Can you work these out from the model? Positions are in its coordinate system, mm. A direction names the side the tool comes from. Give positions to 0.01 mm unless a question says otherwise; leave off trailing zeros. Loops run counter-clockwise (first coordinate to the right, second up) from the corner with the lowest first, then second, coordinate; pieces in that order, holes last. Notation, with made-up numbers: (28, 26) -> (74, 26) arc R21 cw to (74, 48) -> close; hole circle Ø8 at (79, 48.5). An arc over 180 degrees is marked (long way). Use CSV: the item, a comma, the result in double quotes.
Autodesk Inventor part; units mm, degrees
ref_plane "YZ Plane" through (0, 0, 0) normal (1, 0, 0) x (0, 1, 0)
ref_plane "XZ Plane" through (0, 0, 0) normal (0, 1, 0) x (-1, 0, 0)
ref_plane "XY Plane" through (0, 0, 0) normal (0, 0, 1) x (1, 0, 0)
sketch "Sketch1" plane through (0, 0, 0) normal (0, 1, 0) x (-1, 0, 0)
  line L0 (0, 0) -> (177.8, 0)
  line L1 (177.8, 0) -> (177.8, -508)
  line L2 (177.8, -508) -> (0, -508)
  line L3 (0, -508) -> (0, 0)
  line L4 (11.987, 4.1955) -> (189.787, -503.8045)
  line L5 (-11.987, -4.1955) -> (165.813, -512.1955)
  line L6 (0, -38.444) -> (164.3446, -508)
  line L7 (177.8, -469.556) -> (13.4554, 0)
  line L8 (-11.987, -4.1955) -> (11.987, 4.1955)
  line L9 (189.787, -503.8045) -> (165.813, -512.1955)
  line L10 (0, 0) -> (2.0977, -5.9935)
  circle A0 centre (2.0977, -5.9935) radius 2.032
  line L11 (2.0977, -5.9935) -> (10.4886, -29.9675)
  circle A1 centre (10.4886, -29.9675) radius 2.032
  line L12 (10.4886, -29.9675) -> (18.8795, -53.9415)
  circle A2 centre (18.8795, -53.9415) radius 2.032
  line L13 (18.8795, -53.9415) -> (27.2704, -77.9155)
  circle A3 centre (27.2704, -77.9155) radius 2.032
  line L14 (27.2704, -77.9155) -> (35.6613, -101.8895)
  circle A4 centre (35.6613, -101.8895) radius 2.032
  line L15 (35.6613, -101.8895) -> (177.8, -508)
  line L16 (27.2704, -77.9155) -> (35.6613, -101.8895)
  circle A5 centre (35.6613, -101.8895) radius 2.032
  line L17 (35.6613, -101.8895) -> (44.0522, -125.8635)
  circle A6 centre (44.0522, -125.8635) radius 2.032
  line L18 (35.6613, -101.8895) -> (44.0522, -125.8635)
  circle A7 centre (44.0522, -125.8635) radius 2.032
  line L19 (44.0522, -125.8635) -> (52.4431, -149.8375)
  circle A8 centre (52.4431, -149.8375) radius 2.032
  line L20 (44.0522, -125.8635) -> (52.4431, -149.8375)
  circle A9 centre (52.4431, -149.8375) radius 2.032
  line L21 (52.4431, -149.8375) -> (60.834, -173.8115)
  circle A10 centre (60.834, -173.8115) radius 2.032
  line L22 (52.4431, -149.8375) -> (60.834, -173.8115)
  circle A11 centre (60.834, -173.8115) radius 2.032
  line L23 (60.834, -173.8115) -> (69.2249, -197.7855)
  circle A12 centre (69.2249, -197.7855) radius 2.032
  line L24 (60.834, -173.8115) -> (69.2249, -197.7855)
  circle A13 centre (69.2249, -197.7855) radius 2.032
  line L25 (69.2249, -197.7855) -> (77.6158, -221.7595)
  circle A14 centre (77.6158, -221.7595) radius 2.032
  line L26 (69.2249, -197.7855) -> (77.6158, -221.7595)
  circle A15 centre (77.6158, -221.7595) radius 2.032
  line L27 (77.6158, -221.7595) -> (86.0067, -245.7335)
  circle A16 centre (86.0067, -245.7335) radius 2.032
  line L28 (77.6158, -221.7595) -> (86.0067, -245.7335)
  circle A17 centre (86.0067, -245.7335) radius 2.032
  line L29 (86.0067, -245.7335) -> (94.3976, -269.7075)
  circle A18 centre (94.3976, -269.7075) radius 2.032
  line L30 (86.0067, -245.7335) -> (94.3976, -269.7075)
  circle A19 centre (94.3976, -269.7075) radius 2.032
  line L31 (94.3976, -269.7075) -> (102.7885, -293.6815)
  circle A20 centre (102.7885, -293.6815) radius 2.032
  line L32 (94.3976, -269.7075) -> (102.7885, -293.6815)
  circle A21 centre (102.7885, -293.6815) radius 2.032
  line L33 (102.7885, -293.6815) -> (111.1794, -317.6555)
  circle A22 centre (111.1794, -317.6555) radius 2.032
  line L34 (102.7885, -293.6815) -> (111.1794, -317.6555)
  circle A23 centre (111.1794, -317.6555) radius 2.032
  line L35 (111.1794, -317.6555) -> (119.5703, -341.6295)
  circle A24 centre (119.5703, -341.6295) radius 2.032
  line L36 (111.1794, -317.6555) -> (119.5703, -341.6295)
  circle A25 centre (119.5703, -341.6295) radius 2.032
  line L37 (119.5703, -341.6295) -> (127.9612, -365.6035)
  circle A26 centre (127.9612, -365.6035) radius 2.032
  line L38 (119.5703, -341.6295) -> (127.9612, -365.6035)
  circle A27 centre (127.9612, -365.6035) radius 2.032
  line L39 (127.9612, -365.6035) -> (136.3521, -389.5775)
  circle A28 centre (136.3521, -389.5775) radius 2.032
  line L40 (127.9612, -365.6035) -> (136.3521, -389.5775)
  circle A29 centre (136.3521, -389.5775) radius 2.032
  line L41 (136.3521, -389.5775) -> (144.743, -413.5515)
  circle A30 centre (144.743, -413.5515) radius 2.032
  line L42 (136.3521, -389.5775) -> (144.743, -413.5515)
  circle A31 centre (144.743, -413.5515) radius 2.032
  line L43 (144.743, -413.5515) -> (153.1339, -437.5255)
  circle A32 centre (153.1339, -437.5255) radius 2.032
  line L44 (144.743, -413.5515) -> (153.1339, -437.5255)
  circle A33 centre (153.1339, -437.5255) radius 2.032
  line L45 (153.1339, -437.5255) -> (161.5248, -461.4995)
  circle A34 centre (161.5248, -461.4995) radius 2.032
  line L46 (153.1339, -437.5255) -> (161.5248, -461.4995)
  circle A35 centre (161.5248, -461.4995) radius 2.032
  line L47 (161.5248, -461.4995) -> (169.9157, -485.4735)
  circle A36 centre (169.9157, -485.4735) radius 2.032
  dimension "d0" = 177.8
  dimension "d1" = 508
  dimension "d19" = 25.4
extrude "Extrusion1" add sketch "Sketch1" against normal blind 25.4 contours L8 L4 L0 | L10 A0 L11 A1 L12 A2 L13 A3 L14 A4 L15 A6 A8 A10 A12 A14 A16 A18 A20 A22 A24 A26 A28 A30 A32 A34 A36 L2 L5 L3 | L0 L4 L1 L15 A36 A34 A32 A30 A28 A26 A24 A22 A20 A18 A16 A14 A12 A10 A8 A6 A4 L14 A3 L13 A2 L12 A1 L11 A0 L10
sketch "Sketch3" plane through (-11.987, -25.4, 4.1955) normal (0.3304, 0, 0.9439) x (0.9439, 0, -0.3304)
  line L0 (0, 25.4) -> (0, 0)
  line L1 (25.4, 25.4) -> (25.4, 0)
  line L2 (0, 25.4) -> (25.4, 25.4)
  line L3 (25.4, 25.4) -> (25.4, 0)
  line L4 (25.4, 0) -> (0, 0)
  line L5 (0, 0) -> (0, 25.4)
  line L6 (0, 25.4) -> (2.54, 25.4)
  line L7 (0, 25.4) -> (12.7, 25.4)
  line L8 (25.4, 0) -> (22.86, 0)
  line L9 (25.4, 0) -> (12.7, 0)
  line L10 (2.54, 25.4) -> (22.86, 25.4)
  line L11 (22.86, 0) -> (2.54, 0)
  line L12 (2.54, 25.4) -> (2.54, 22.86)
  line L13 (22.86, 0) -> (22.86, 2.54)
  line L14 (2.54, 22.86) -> (22.86, 22.86)
  line L15 (22.86, 22.86) -> (22.86, 2.54)
  line L16 (22.86, 2.54) -> (2.54, 2.54)
  line L17 (2.54, 2.54) -> (2.54, 22.86)
  dimension "d23" = 25.4
  dimension "d24" = 25.4
  dimension "d25" = 2.54
  dimension "d26" = 2.54
  dimension "d27" = 2.54
  dimension "d28" = 2.54
extrude "Extrusion2" cut sketch "Sketch3" against normal blind 556.26 contours L14 L15 L16 L17
extrude "Extrusion3" cut sketch "Sketch1" against normal blind 25.4 contours L8 L4 L0
properties part number "1 x 1 x 0.100 Pre-drilled stock ( angled)"
(1) Will these pins go through, and if not, where does the flat tip stop? pin 1 Ø2.5 at (x, z) = (-52.44, -149.84) entering from +Y; pin 2 Ø4 at (y, z) = (-2.5, -250.5) entering from +X.
Answer sheet:
pin 1,"passes through"
pin 2,"stops at x = -73.52"
(2) If we section it at B-B, the plane z = -212: Write out the boundary of the cut face in (x, y), then the cut area to 3 significant figures.
Answer sheet:
outline,"(-87.66, -25.4) -> (-60.74, -25.4) -> (-60.74, 0) -> (-87.66, 0) -> close; hole (-84.97, -22.86) -> (-63.44, -22.86) -> (-63.44, -2.54) -> (-84.97, -2.54) -> close"
area,"246 mm2"
(3) If we section it at A-A, the plane y = -17.5: Write out the boundary of the cut face in (x, z).
Answer sheet:
outline,"(-177.8, -477.19) -> (-10.76, 0) -> (-13.46, 0) -> (-177.8, -469.56) -> close; (-167.05, -508) -> (-164.34, -508) -> (0, -38.44) -> (0, -30.75) -> close"
(4) If I drill on L1, parallel to Y at x = -98, z = -299; L2, parallel to X at y = -6.25, z = -459; L3, parallel to X at y = -7.5, z = -255, over which ranges is the centre line in solid material (lowest first)? Write a range as from..to.
Answer sheet:
L1,"y = -25.4..-22.86, -2.54..0"
L2,"x = -174.11..-171.43, -149.9..-147.19"
L3,"x = -102.71..-100.02, -78.5..-75.79"
(5) We'd pull the mould along Y, two halves only. Please class faces 1 (the face through (-88, 0, -253)), 2 (the face through (-82.36, -12.56, -266.04)), 3 (the face through (0, -13, -32)): released by +Y, released by -Y, zero draft, split by the parting line, or undercut.
Answer sheet:
face 1,"released by +Y"
face 2,"undercut"
face 3,"zero draft"
(6) Which directions (+Z, -Z, +X, -X, +Y, -Y) give clear straight access to the entire face, cutting with the end or side of a thin tool? Please do faces 4 (the face through (-88, -2.54, -250)), 5 (the face through (-166.7, -12.5, -508)).
Answer sheet:
face 4,"none"
face 5,"-Z, +X, -X, +Y, -Y"
